CAD build for the part. Positions are in the model's coordinates, mm. A direction names the side the tool comes from. Coordinates: 2 decimals unless noted, no trailing zeros. Write each question's results on one line, items separated by ' | '. Start each with the question number.
Q1. Which spindle directions (+Z, -Z, +X, -X, +Y, -Y) get a long thin tool onto all of the face, cutting with end or side? Do faces 4 (the cylindrical face through (5.5, -49.17, 18.92)), 5 (the cylindrical face through (9.5, 0.01, 12.69)), 6 (the flat face through (0, -48.763, 13)). Say none if no direction does.
Q2. Band-saw the part on A-A, the plane y = -31. Count the separate pieces of the cut face and the enclosed holes in it, then the cut area to 3 significant figures.
Q3. Wall check: probe 1 along Z at (x, y) = (-12.5, -49.2); probe 2 along X at (y, z) = (-35, 23.5); probe 3 along Y at (x, z) = (37, 1.75). Give the ranges that are in metal, low to high.
Q4. Pin check, flat tips, straight feed: P1, Ø4, axis at y = 21, z = 8, coming from the -X side; P2, Ø1, axis at x = 28.5, z = 7.5, coming from the +Y side; P3, Ø5, axis at y = -25.5, z = 16.5, coming from the +X side; P4, Ø3, axis at x = 20.5, y = 31, coming from the -Z side. Stop position of each tip, or through.
Q5. Pull direction Y, two halves, no side cores. Call faces 1 (the flat face through (43.12, -24.44, 12.68)), 2 (the flat face through (24, 0, 0)), 3 (the cylindrical face through (21.38, 37.04, 21.92)): released by +Y, released by -Y, zero draft, split by the parting line, or undercut.
```python
from build123d import *

# Parameters (mm, degrees)
SKETCH_R              = 9.5
PAD_DEPTH             = 0.4
POLARPATTERN_COUNT    = 6
PAD001_DEPTH          = 25
POLARPATTERN001_COUNT = 3
POLARPATTERN001_ANGLE = 120
SKETCH002_R           = 9.5
POCKET_DEPTH          = 2
POLARPATTERN002_COUNT = 6
SKETCH003_R           = 1.5
PAD002_DEPTH          = 25
POCKET001_DEPTH       = 25


with BuildPart() as part:
    # Sketch → Pad (new body, symmetric)
    with BuildSketch(Plane.XZ):
        with BuildLine():
            Line((0, 0), (57, 0))
            Line((57, 0), (57, 25))
            Line((57, 25), (0, 25))
            Line((0, 25), (0, 22))
            ThreePointArc((0, 3), (9.5, 12.5), (0, 22))
            Line((0, 3), (0, 0))
        make_face()
        with Locations((22, 12.5)):
            Circle(SKETCH_R, mode=Mode.SUBTRACT)
        with Locations((44, 12.5)):
            Circle(SKETCH_R, mode=Mode.SUBTRACT)
    pad = extrude(amount=PAD_DEPTH, both=True)

    # PolarPattern: Pad ×6 about axis
    polarpattern_axis = Axis((0, 0, 0), (0, 0, 1))
    for i in range(1, POLARPATTERN_COUNT):
        add(pad.rotate(polarpattern_axis, i * 360 / POLARPATTERN_COUNT))

    # Sketch001 (on Face61 of PolarPattern) → Pad001 (join)
    with BuildSketch(Plane(origin=(0, 0, 25), x_dir=(-1, 0, 0), z_dir=(0, 0, 1))):
        Polygon((-28.15359, 49.563448), (28.15359, 49.563448), (27.69171, 48.763448), (-27.69171, 48.763448), align=None)
    pad001 = extrude(amount=-PAD001_DEPTH)

    # PolarPattern001: Pad001 ×3 about axis
    polarpattern001_axis = Axis((0, 0, 25), (0, 0, 1))
    for i in range(1, POLARPATTERN001_COUNT):
        add(pad001.rotate(polarpattern001_axis, i * POLARPATTERN001_ANGLE / (POLARPATTERN001_COUNT - 1)))

    # Sketch002 (on Face59 of Pad001) → Pocket (cut)
    with BuildSketch(Plane.XZ.offset(49.563448)):
        with Locations((-12.5, 12.5)):
            Circle(SKETCH002_R)
        with Locations((12.5, 12.5)):
            Circle(SKETCH002_R)
    pocket = extrude(amount=-POCKET_DEPTH, mode=Mode.SUBTRACT)

    # PolarPattern002: Pocket ×6 about axis
    polarpattern002_axis = Axis((0, 0, 0), (0, 0, 1))
    for i in range(1, POLARPATTERN002_COUNT):
        add(pocket.rotate(polarpattern002_axis, i * 360 / POLARPATTERN002_COUNT), mode=Mode.SUBTRACT)

    # Sketch003 (on Face68 of PolarPattern002) → Pad002 (join)
    with BuildSketch(Plane(origin=(0, 0, 25), x_dir=(-1, 0, 0), z_dir=(0, 0, 1))):
        Circle(SKETCH003_R)
    extrude(amount=-PAD002_DEPTH)

    # Sketch004 (on Face83 of Pad002) → Pocket001 (cut)
    with BuildSketch(Plane(origin=(0, 0, 25), x_dir=(-1, 0, 0), z_dir=(0, 0, 1))):
        Polygon((28.84641, 49.163448), (-28.15359, -49.563448), (31.376045, -54.075596), (79.795143, 24.207651), align=None)
    extrude(amount=-POCKET001_DEPTH, mode=Mode.SUBTRACT)


solid = part.part
```
Results below:
1) face 4: -Y | face 5: none | face 6: +Z, -Z
2) separate pieces: 6 | enclosed holes: 0 | area: 36.8 mm²
3) probe 1: z = 0 to 3, 22 to 25 | probe 2: x = -20.67 to -19.75, 19.75 to 20.67, 36.1 to 37.02 | probe 3: y = -35.04 to -33.44, -0.4 to 0.4, 33.44 to 35.04
4) P1: stops at x = 43.03 | P2: stops at y = 49.56 | P3: stops at x = 43.95 | P4: passes through
5) face 1: released by -Y | face 2: zero draft | face 3: undercut
